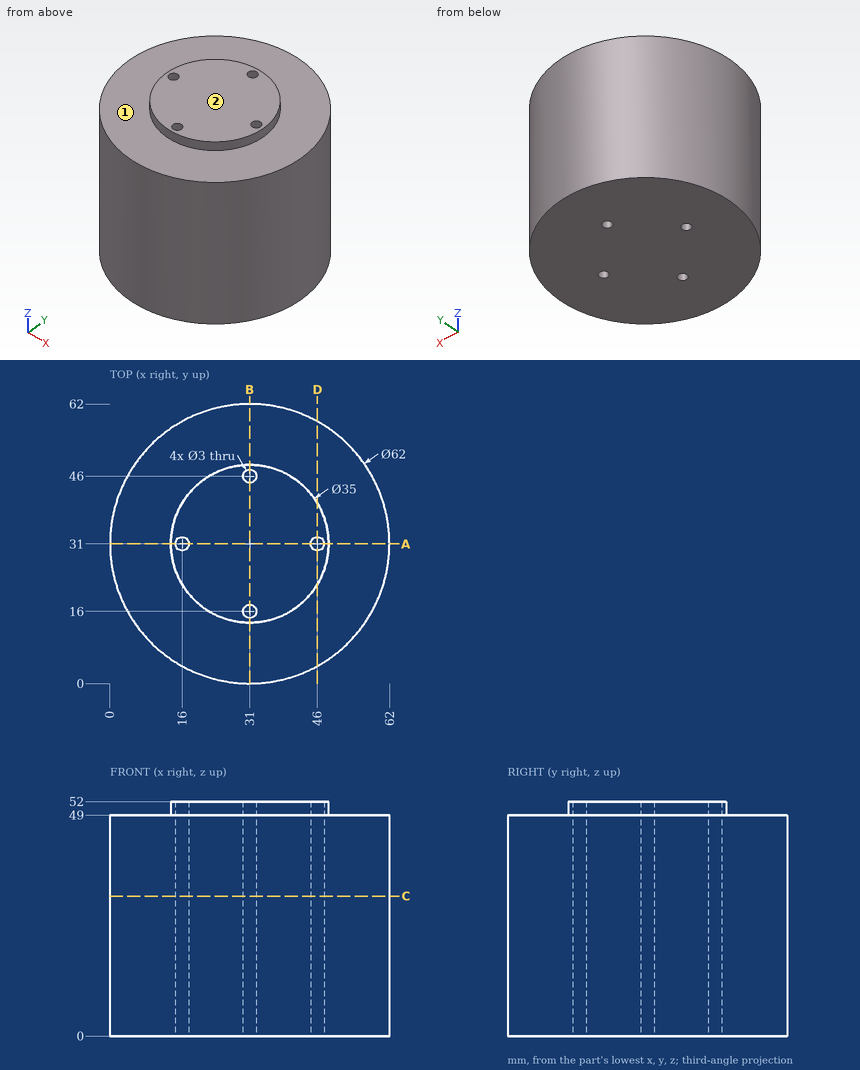
Job drawing, mm, ordinate dimensions from the low corner. One solid piece. A direction names the side the tool comes from. Give positions to 0.01 mm unless a question says otherwise; leave off trailing zeros. Loops run counter-clockwise (first coordinate to the right, second up) from the corner with the lowest first, then second, coordinate; pieces in that order, holes last. Notation, with made-up numbers: M 57,69 L 70,69 A24 cw 70,88 Z; hole C 77.5,31 d4. An arc over 180 degrees is marked long. Answer in a Markdown table with one row per item. Add a question column.
Item 1: Drop flat-ended pins along their axis: P1, Ø2.5, axis at x = 46, y = 31, coming from the -Z side; P2, Ø10, axis at x = 35, z = 29, coming from the -Y side; P3, Ø2, axis at y = 43.5, z = 19.5, coming from the +X side; P4, Ø8, axis at y = 48.5, z = 22.5, coming from the -X side. Give the stop position or say it passes through.
Item 2: Band-saw the part on D-D on x = 46. Give the cut face in (y, z).
Item 3: Probe probe 1 along Y at (x, z) = (31, 18.5); probe 2 along Z at (x, y) = (15, 15); probe 3 along Y at (x, z) = (46, 20). List the from-to ranges inside material, lowest first.
Item 4: Band-saw the part on C-C on z = 31. Give the cut face in (x, y).
Item 5: Band-saw the part on A-A on y = 31. Give the cut face in (x, z), then the cut area to 3 significant figures.
Item 6: Tool access for the marked faces 1 and 2: list every direction of +Z, -Z, +X, -X, +Y, -Y with a clear straight run to the whole face (end or side of a thin tool).
Reply:
| question | item | result |
|---|---|---|
| 1 | P1 | passes through |
| 1 | P2 | stops at y = 0 |
| 1 | P3 | stops at x = 59.79 |
| 1 | P4 | stops at x = 3.09 |
| 2 | outline | M 3.87,0 L 29.5,0 L 29.5,52 L 21.99,52 L 21.99,49 L 3.87,49 Z; M 32.5,0 L 58.13,0 L 58.13,49 L 40.01,49 L 40.01,52 L 32.5,52 Z |
| 3 | probe 1 | y = 0 to 14.5, 17.5 to 44.5, 47.5 to 62 |
| 3 | probe 2 | z = 0 to 49 |
| 3 | probe 3 | y = 3.87 to 29.5, 32.5 to 58.13 |
| 4 | outline | C 31,31 d62; hole C 16,31 d3; hole C 31,16 d3; hole C 31,46 d3; hole C 46,31 d3 |
| 5 | outline | M 0,0 L 14.5,0 L 14.5,52 L 13.5,52 L 13.5,49 L 0,49 Z; M 17.5,0 L 44.5,0 L 44.5,52 L 17.5,52 Z; M 47.5,0 L 62,0 L 62,49 L 48.5,49 L 48.5,52 L 47.5,52 Z |
| 5 | area | 2,830 mm^2 |
| 6 | face 1 | +Z |
| 6 | face 2 | +Z, +X, -X, +Y, -Y |
